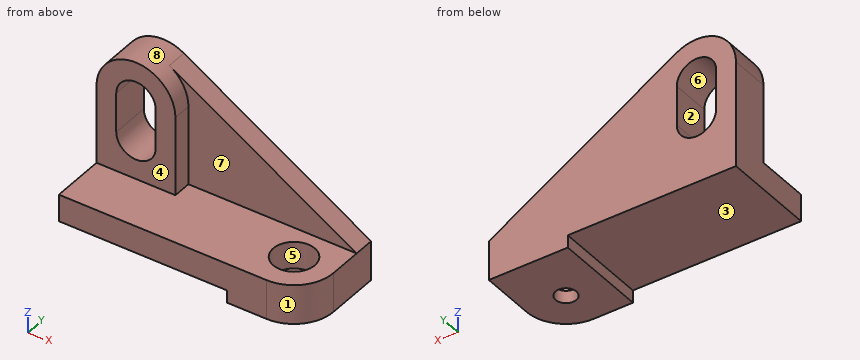
Autodesk Fusion 360 part; units mm, degrees
sketch "Sketch1" plane through (0, 0, 0) normal (0, 1, 0) x (1, 0, 0)
  line L0 (0, 0) -> (38, 0)
  line L1 (38, 0) -> (38, -38)
  line L2 (38, -38) -> (0, -38)
  line L3 (0, -38) -> (0, 0)
  circle A0 centre (19, -38) radius 19
  line L4 (9.5, -38) -> (28.5, -38)
  line L5 (28.5, -38) -> (28.5, -19)
  line L6 (28.5, -19) -> (9.5, -19)
  line L7 (9.5, -19) -> (9.5, -38)
  circle A1 centre (19, -38) radius 9.5
  circle A2 centre (19, -19) radius 9.5
  dimension "d1" = 38
  dimension "d2" = 38
  dimension "d3" = 19
  dimension "d4" = 19
  dimension "d5" = 19
  dimension "d6" = 9.5
extrude "Extrude1" add sketch "Sketch1" along normal blind 19 contours L0 L1 L3 A0 L5 L7 A2 | L2 A0 L7 | L2 A0 A1 | L2 A0 L5 makes body 1
sketch "Sketch1 (2)" plane through (0, 19, 0) normal (0, 1, 0) x (-1, 0, 0) in component "sideline"
  arc A0 (-28.5, 19) -> (-9.5, 19) centre (-19, 19) ccw
  line L0 (-28.5, 19) -> (-28.5, 38)
  arc A1 (-9.5, 38) -> (-28.5, 38) centre (-19, 38) ccw
  line L1 (-9.5, 38) -> (-9.5, 19)
  arc A2 (0, 38) -> (-38, 38) centre (-19, 38) ccw
  line L2 (-38, 38) -> (-38, 0)
  line L3 (-38, 0) -> (0, 0)
  line L4 (0, 0) -> (0, 38)
  line L5 (-38, 0) -> (-119, 0)
  line L6 (-119, 0) -> (-28.7963, 54.2798)
  dimension "d9" = 81
extrude "Extrude1'" add sketch "Sketch1 (2)" against normal blind 10 separate body contours A2 L2 L5 L6 makes body 2 in component "sideline"
combine "Combine1" operation add target body 2 tool bodies 1 in component "sideline"
sketch "Sketch2" plane through (0, 0, 0) normal (0, 0, 1) x (1, 0, 0) in component "sideline"
  line L0 (119, 19) -> (0, 19)
  line L1 (0, 19) -> (0, -26)
  line L2 (0, -26) -> (100, -26)
  line L3 (119, -7) -> (119, 19)
  line L4 (113.8585, -7) -> (125, -7)
  circle A0 centre (100, -7) radius 10
  circle A1 centre (100, -7) radius 5
  arc A2 (100, -26) -> (119, -7) centre (100, -7) ccw
  line L5 (100, -7) -> (100, -33.6154)
  line L6 (100, -26) -> (91, -26)
  line L7 (100, -26) -> (81, -26)
  line L8 (81, -26) -> (81, 19)
  dimension "d19" = 19
extrude "Extrude2" add sketch "Sketch2" against normal blind 13 contours L0 L2 L3 A2 L6 L7 L8 | L0 L1 L2 L8 bodies 2 in component "sideline"
sketch "Sketch3" plane through (0, 0, -13) normal (0, 0, -1) x (1, 0, 0) in component "sideline"
  circle A0 centre (100, 7) radius 10
  line L0 (119, -19) -> (119, 7)
  arc A1 (119, 7) -> (100, 26) centre (100, 7) ccw
  line L1 (100, 26) -> (0, 26)
  line L2 (0, 26) -> (0, -19)
  line L3 (0, -19) -> (119, -19)
  circle A2 centre (100, 7) radius 5
  line L4 (80.9955, 26) -> (80.9955, -19)
  dimension "d22" = 10
extrude "Extrude3" add sketch "Sketch3" along normal blind 6 contours A0 | L0 A1 L1 L3 L4 bodies 2 in component "sideline"
component "sideline" placed x (1, 0, 0) y (0, 1, 0) z (0, 0, 1) at (0, 0, 0)
The listing builds one solid part. Answer for the finished solid, in the listing's coordinates (mm). Face numbers are marked on the shaded views. A direction names the side the tool comes from. Coordinates: 2 decimals unless noted, no trailing zeros. Order: outer loops, then holes, each group sorted by start corner. A loop starts at its lowest first (then second) coordinate and runs counter-clockwise, first axis right, second up. Notation, with made-up numbers: M 6,64 L 19,64 A33 ccw 19,93 Z; hole C 7.5,61 d3. An arc over 180 degrees is marked long. Answer as a JSON object with one key per item and string values. Group by question number.
1. Straight lines are drawn through the part: line 1 (X direction, y = -7, z = -3); line 2 (Y direction, x = 100, z = -16.95); line 3 (Y direction, x = 100, z = -5.75). For each, find the intervals that lie inside material, in ascending order.
2. Section C-C on y = -5.5 is taken. Write down the section's boundary in (x, z), then the cut area to 3 significant figures.
3. Determine the mould class of the marked faces 1, 2 and 3 for opening direction X: released by +X, released by -X, zero draft, split by the parting line, or undercut.
4. Section B-B on x = 19 is taken. Write down the section's boundary in (y, z).
5. A tool of negligible diameter and unlimited length cuts with its end or side. For the marked faces 4, 5, 6, 7 and 8, from which of +Z, -Z, +X, -X, +Y, -Y can it reach the whole face along a straight path? Write none if from no direction.
6. Section A-A on z = 12 is taken. Write down the section's boundary in (x, y).
7. Section D-D on z = -8 is taken. Write down the section's boundary in (x, y), then the cut area to 3 significant figures.
8. Flat-ended cylindrical pins translate along their axes: P1, Ø16.5, axis at x = 87, z = 21, coming from the -Y side; P2, Ø6, axis at y = -15.5, z = -1, coming from the +X side; P3, Ø1, axis at x = 37, z = 12.5, coming from the -Y side. Find the tip coordinate at first contact, or state that the pin passes through.
Values follow:
{
 "1": {"line 1": "0 to 90, 110 to 119", "line 2": "-26 to -12, -2 to 19", "line 3": "-26 to -17, 3 to 19"},
 "2": {"outline": "M 0,-13 L 81,-13 L 81,-19 L 95.23,-19 L 95.23,-13 L 90.11,-13 L 90.11,0 L 0,0 Z; M 104.77,-19 L 119,-19 L 119,0 L 109.89,0 L 109.89,-13 L 104.77,-13 Z", "area": "1,460 mm2"},
 "3": {"face 1": "released by +X", "face 2": "undercut", "face 3": "zero draft"},
 "4": {"outline": "M -26,-13 L 19,-13 L 19,9.5 L 0,9.5 L 0,0 L -26,0 Z; M 0,47.5 L 19,47.5 L 19,57 L 0,57 Z"},
 "5": {"face 4": "+Z, +X, -X, -Y", "face 5": "+Z", "face 6": "+Y, -Y", "face 7": "+Z, +X, -Y", "face 8": "+Z, -Y"},
 "6": {"outline": "M 0,0 L 12.58,0 L 12.58,19 L 0,19 Z; M 25.42,0 L 38,0 L 38,9 L 99.06,9 L 99.06,19 L 25.42,19 Z"},
 "7": {"outline": "M 0,-26 L 100,-26 A19 ccw 119,-7 L 119,19 L 0,19 Z; hole C 100,-7 d20", "area": "4,960 mm2"},
 "8": {"P1": "y = 9", "P2": "x = 118.19", "P3": "y = 0"}
}
